Read the model definition and answer for the solid it produces. Units are mm, in the model's axes. A direction names the side the tool comes from. Give positions to 0.01 mm unless a question says otherwise; leave off trailing zeros. Order: outer loops, then holes, each group sorted by start corner. A loop starts at its lowest first (then second) coordinate and runs counter-clockwise, first axis right, second up. Notation, with made-up numbers: M -23,20 L 20,20 A33 cw 20,55 Z; hole C -36,21 d7. An arc over 180 degrees is marked long. One line per item, written item: value.
from build123d import *

# Parameters (mm, degrees)
CUTSKETCH_W             = 9
CUTSKETCH_H             = 22
BOLTCIRCLEPATTERN_COUNT = 4


with BuildPart() as part:
    # BaseSketch → BaseRevolve (revolve)
    with BuildSketch(Plane.XY, mode=Mode.PRIVATE) as baserevolve_sk:
        Polygon((-31.75, 0), (-31.75, -45), (-59, -45), (-59, -29), (-92.5, -29), (-92.5, -9), (-48, -9), (-48, -23), (-54, -29), (-46, -29), (-38.05, -10), (-38.05, -3.637306696), align=None)
    revolve(baserevolve_sk.sketch.rotate(Axis((0, 0, 0), (0, -1, 0)), 270), axis=Axis((0, 0, 0), (0, -1, 0)))

    # CutSketch → CenterRevCut (revolve, cut)
    with BuildSketch(Plane.XY, mode=Mode.PRIVATE) as centerrevcut_sk:
        with Locations((-77, -19)):
            Rectangle(CUTSKETCH_W, CUTSKETCH_H)
    centerrevcut = revolve(centerrevcut_sk.sketch.rotate(Axis((-72.5, 10.805368121, 0), (0, -1, 0)), 270), axis=Axis((-72.5, 10.805368121, 0), (0, -1, 0)), mode=Mode.SUBTRACT)

    # BoltCirclePattern: CenterRevCut ×4 about axis
    boltcirclepattern_axis = Axis((0, 0, 0), (0, 1, 0))
    for i in range(1, BOLTCIRCLEPATTERN_COUNT):
        add(centerrevcut.rotate(boltcirclepattern_axis, i * 360 / BOLTCIRCLEPATTERN_COUNT), mode=Mode.SUBTRACT)


solid = part.part
1) Determine the mould class of faces 6 (the face through (1.951, -18.86, -63.714)), 7 (the face through (-9.63, -0.18, 30.58)), 8 (the face through (40, -9, 40)) for opening direction X: +X half, -X half, draft (parallel to the pull), parting line (faces both ways), or undercut.
Reported:
face 6: undercut
face 7: parting line
face 8: draft
2) Each of these flat-tipped pins is pushed along its axis until it touches: pin 1 Ø1.5 at (x, y) = (-59.5, -18.5) entering from +Z; pin 2 Ø3 at (x, z) = (-42, 62) entering from -Y; pin 3 Ø5 at (y, z) = (-9, -68.5) entering from +X. Where does it stop, or does it pass through?
Reported:
pin 1: stops at z = 71.45
pin 2: stops at y = -29
pin 3: stops at x = 64.81
3) Consider probe 1 along X at (y, z) = (-16.5, 0); probe 2 along X at (y, z) = (-18, 0); probe 3 along Y at (x, z) = (-83.5, 6). Determine where each line is inside the solid, lowest interval first.
Reported:
probe 1: x = -92.5 to -81.5, -63.5 to -48, -40.77 to -31.75, 31.75 to 40.77, 48 to 63.5, 81.5 to 92.5
probe 2: x = -92.5 to -81.5, -63.5 to -48, -41.4 to -31.75, 31.75 to 41.4, 48 to 63.5, 81.5 to 92.5
probe 3: y = -29 to -9
4) Which of the six approach directions +Z, -Z, +X, -X, +Y, -Y give full straight-line access (tool end or side, diameter ignored) to faces 1 (the face through (47.225, -23.375, -10.487)), 2 (the face through (63.714, -18.86, 1.951)), 3 (the face through (-42, -29, 42)), 4 (the face through (-32.08, -6.77, 20.46)), 5 (the face through (25, -45, -25))?
Reported:
face 1: none
face 2: +Y, -Y
face 3: -Y
face 4: +Y
face 5: +Z, -Z, +X, -X, -Y
5) Find section B-B, the plane y = -19. Write down the section's boundary in (x, z).
Reported:
outline: C 0,0 d185; C 0,0 d83.63; hole C -72.5,0 d18; hole C 0,0 d96; hole C 0,0 d63.5; hole C 0,-72.5 d18; hole C 0,72.5 d18; hole C 72.5,0 d18
6) Find section A-A, the plane x = 0. Count the separate pieces of the cut face and the enclosed holes in it, plus the area to 3 significant figures.
Reported:
separate pieces: 4
enclosed holes: 0
area: 2,390 mm^2
7) Find section D-D, the plane x = -72.5. Write down the section's boundary in (y, z).
Reported:
outline: M -29,-57.45 L -9,-57.45 L -9,-9 L -29,-9 Z; M -29,9 L -9,9 L -9,57.45 L -29,57.45 Z
